Geometry: see drawing. Coordinates: mm, zero at the bounding-box minimum. Give positions to 0.01 mm unless a question says otherwise; leave off trailing zeros. Write each loop counter-clockwise with the first axis right and the second up, starting at its lowest first coordinate (ties: lowest second). Pieces come first, ordered by that corner, then holes. Notation, with made-up numbers: M 87.5,27.25 L 116.5,27.25 A20 ccw 116.5,51.25 Z; hole C 19,-15.75 d3. An arc over 180 degrees is marked long. Use a Markdown table: item, result. Add a question column.
(1) Cut plane A-A (z = 40). Output: boundary loops of the cut face in (x, y).
(2) Pin query (flat end, axial travel): pin 1 Ø3.5 at (x, z) = (20, 50) entering from -Y; pin 2 Ø4 at (x, z) = (32.5, 20.5) entering from +Y. Return the tip coordinate at first contact, or that it passes through.
(3) Cut plane B-B (y = 55). Output: boundary loops of the cut face in (x, z).
(4) Cut plane C-C (z = 30). Output: boundary loops of the cut face in (x, y).
(5) Draft query along Z for the marked faces 1, 2, 3 and 4. Return one class per face: released by +Z, released by -Z, zero draft, split by the parting line, or undercut.
(6) Material intervals for L1, parallel to Z at x = 60, y = 10.75; L2, parallel to X at y = 15, z = 10; L3, parallel to Y at x = 10, z = 11.75, sorted ascending.
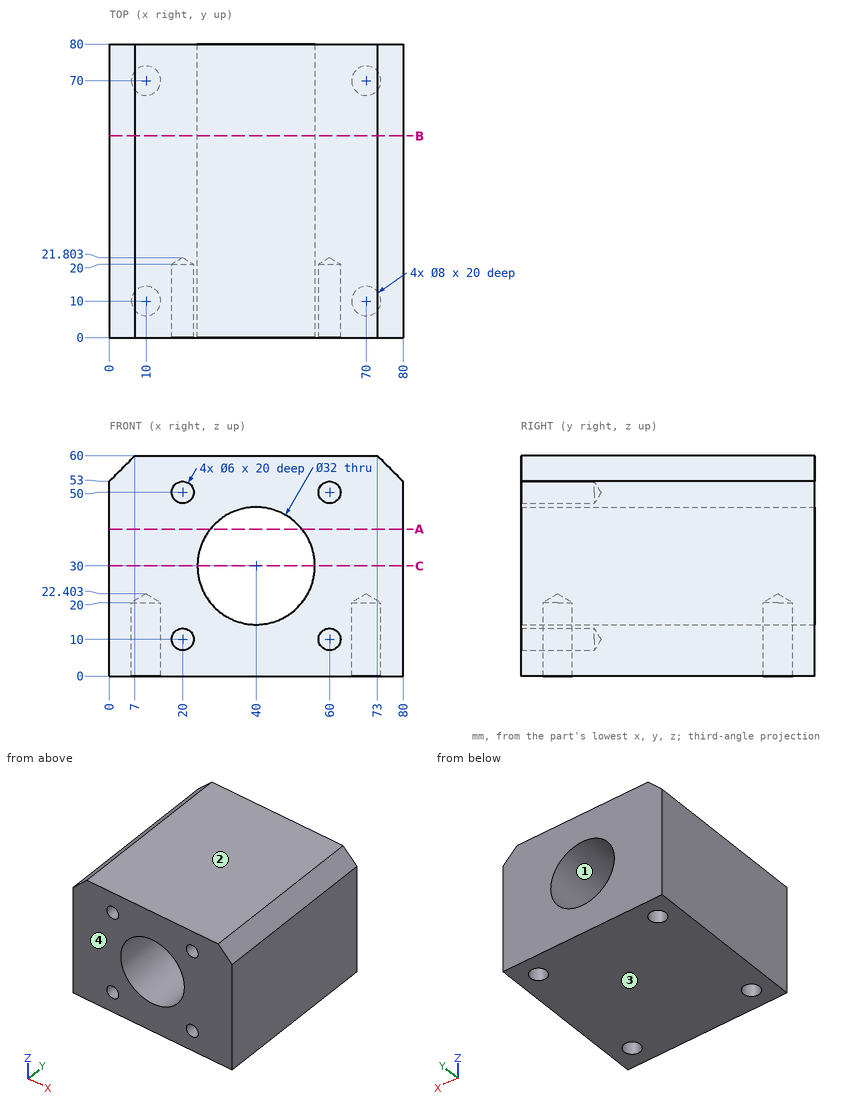
Answer list:
| question | item | result |
|---|---|---|
| 1 | outline | M 0,0 L 27.51,0 L 27.51,80 L 0,80 Z; M 52.49,0 L 80,0 L 80,80 L 52.49,80 Z |
| 2 | pin 1 | y = 20.75 |
| 2 | pin 2 | through |
| 3 | outline | M 0,0 L 80,0 L 80,53 L 73,60 L 7,60 L 0,53 Z; hole C 40,30 d32 |
| 4 | outline | M 0,0 L 24,0 L 24,80 L 0,80 Z; M 56,0 L 80,0 L 80,80 L 56,80 Z |
| 5 | face 1 | undercut |
| 5 | face 2 | released by +Z |
| 5 | face 3 | released by -Z |
| 5 | face 4 | zero draft |
| 6 | L1 | 0 to 7, 13 to 47, 53 to 60 |
| 6 | L2 | 0 to 17, 23 to 57, 63 to 80 |
| 6 | L3 | 0 to 6, 14 to 66, 74 to 80 |
